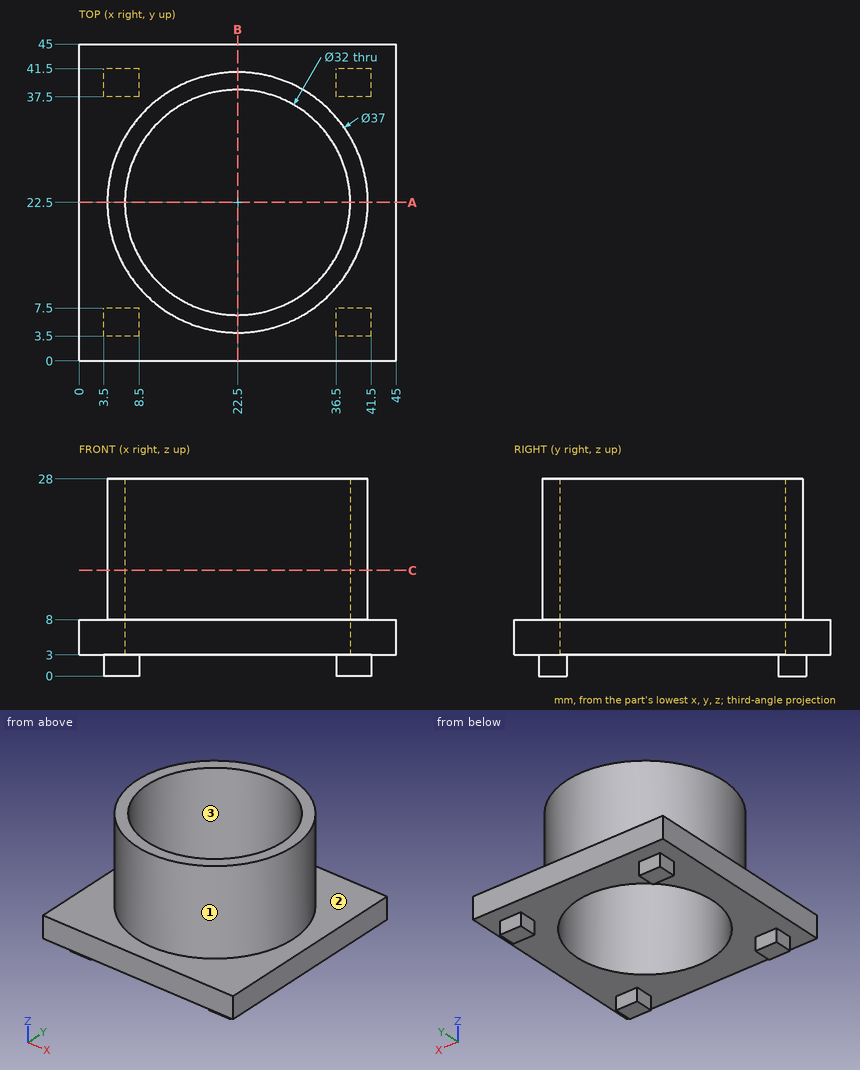
Print and shaded views of the part. All mm, measured from the part's lowest x, y and z. Coordinates: 2 decimals unless noted, no trailing zeros. Loops run counter-clockwise (first coordinate to the right, second up) from the corner with the lowest first, then second, coordinate; pieces in that order, holes last. Notation, with made-up numbers: (40.25, 58.5) -> (68.25, 58.5) arc R13 cw to (68.25, 73.5) -> close; hole circle Ø6 at (32.25, 66). An arc over 180 degrees is marked (long way). Use a Markdown table: item, result. Add a question column.
Item 1: Band-saw the part on C-C on z = 15. Write the cut outline in (x, y).
Item 2: Probe probe 1 along Y at (x, z) = (22.5, 17); probe 2 along X at (y, z) = (23, 17.5); probe 3 along Z at (x, y) = (4, 16.5). List the from-to ranges inside material, lowest first.
Item 3: Flat gauge pins, fed straight in: P1, Ø2.5, axis at x = 39, z = 1, coming from the +Y side; P2, Ø6, axis at x = 33.5, z = 23, coming from the -Y side; P3, Ø12, axis at x = 23.5, y = 36.5, coming from the -Z side; P4, Ø19, axis at x = 22.5, y = 22.5, coming from the -Z side. Where does each tip first touch, or does it go through?
Item 4: Pull direction Y, two halves, no side cores. Call the marked faces 1, 2 and 3: +Y half, -Y half, draft (parallel to the pull), parting line (faces both ways), or undercut.
Item 5: Band-saw the part on A-A on y = 22.5. Write the cut outline in (x, z).
Geometry says:
| question | item | result |
|---|---|---|
| 1 | outline | circle Ø37 at (22.5, 22.5); hole circle Ø32 at (22.5, 22.5) |
| 2 | probe 1 | 4 to 6.5, 38.5 to 41 |
| 2 | probe 2 | 4.01 to 6.51, 38.49 to 40.99 |
| 2 | probe 3 | 3 to 8 |
| 3 | P1 | y = 41.5 |
| 3 | P2 | y = 5.82 |
| 3 | P3 | z = 3 |
| 3 | P4 | through |
| 4 | face 1 | parting line |
| 4 | face 2 | draft |
| 4 | face 3 | undercut |
| 5 | outline | (0, 3) -> (6.5, 3) -> (6.5, 28) -> (4, 28) -> (4, 8) -> (0, 8) -> close; (38.5, 3) -> (45, 3) -> (45, 8) -> (41, 8) -> (41, 28) -> (38.5, 28) -> close |
